from build123d import *

# Parameters (mm, degrees)
F0_R     = 9.283405223
F1_DEPTH = 25.4
F2_SIZE  = 5
F3_SIZE  = 5


with BuildPart() as f1:
    # F0 (on Top) → F1 (new body)
    with BuildSketch(Plane.XY):
        Polygon((-17.8308878342, 27.9613517337), (-33.1306848427, -1.4613259696), (-15.2997970084, -29.4226777033), (17.8308878342, -27.9613517337), (33.1306848427, 1.4613259696), (15.2997970084, 29.4226777033), align=None)
        Circle(F0_R, mode=Mode.SUBTRACT)
    extrude(amount=F1_DEPTH)

    # F2
    f2_edges = [f1.edges().sort_by_distance(p)[0] for p in [
        (-17.830888, 27.961352, 12.7),
        (15.299797, 29.422678, 12.7),
        (33.130685, 1.461326, 12.7),
        (-33.130685, -1.461326, 12.7),
        (-15.299797, -29.422678, 12.7),
        (17.830888, -27.961352, 12.7),
    ]]
    chamfer(f2_edges, length=F2_SIZE)

    # F3 (call 1 of 12: OpenCascade refuses the feature's edges together)
    f3_edges = [f1.edges().sort_by_distance(p)[0] for p in [
        (24.215241, 15.442002, 0),
    ]]
    chamfer(f3_edges, length=F3_SIZE)

    # F3#2 (call 2 of 12)
    f3_2_edges = [f1.edges().sort_by_distance(p)[0] for p in [
        (-1.265545, 28.692015, 0),
    ]]
    chamfer(f3_2_edges, length=F3_SIZE)

    # F3#3 (call 3 of 12)
    f3_3_edges = [f1.edges().sort_by_distance(p)[0] for p in [
        (24.215241, 15.442002, 25.4),
    ]]
    chamfer(f3_3_edges, length=F3_SIZE)

    # F3#4 (call 4 of 12)
    f3_4_edges = [f1.edges().sort_by_distance(p)[0] for p in [
        (-1.265545, 28.692015, 25.4),
    ]]
    chamfer(f3_4_edges, length=F3_SIZE)

    # F3#5 (call 5 of 12)
    f3_5_edges = [f1.edges().sort_by_distance(p)[0] for p in [
        (-25.480786, 13.250013, 25.4),
    ]]
    chamfer(f3_5_edges, length=F3_SIZE)

    # F3#6 (call 6 of 12)
    f3_6_edges = [f1.edges().sort_by_distance(p)[0] for p in [
        (-25.480786, 13.250013, 0),
    ]]
    chamfer(f3_6_edges, length=F3_SIZE)

    # F3#7 (call 7 of 12)
    f3_7_edges = [f1.edges().sort_by_distance(p)[0] for p in [
        (-24.215241, -15.442002, 25.4),
    ]]
    chamfer(f3_7_edges, length=F3_SIZE)

    # F3#8 (call 8 of 12)
    f3_8_edges = [f1.edges().sort_by_distance(p)[0] for p in [
        (-24.215241, -15.442002, 0),
    ]]
    chamfer(f3_8_edges, length=F3_SIZE)

    # F3#9 (call 9 of 12)
    f3_9_edges = [f1.edges().sort_by_distance(p)[0] for p in [
        (25.480786, -13.250013, 25.4),
    ]]
    chamfer(f3_9_edges, length=F3_SIZE)

    # F3#10 (call 10 of 12)
    f3_10_edges = [f1.edges().sort_by_distance(p)[0] for p in [
        (25.480786, -13.250013, 0),
    ]]
    chamfer(f3_10_edges, length=F3_SIZE)

    # F3#11 (call 11 of 12)
    f3_11_edges = [f1.edges().sort_by_distance(p)[0] for p in [
        (1.265545, -28.692015, 0),
    ]]
    chamfer(f3_11_edges, length=F3_SIZE)

    # F3#12 (call 12 of 12)
    f3_12_edges = [f1.edges().sort_by_distance(p)[0] for p in [
        (1.265545, -28.692015, 25.4),
    ]]
    chamfer(f3_12_edges, length=F3_SIZE)


solid = f1.part
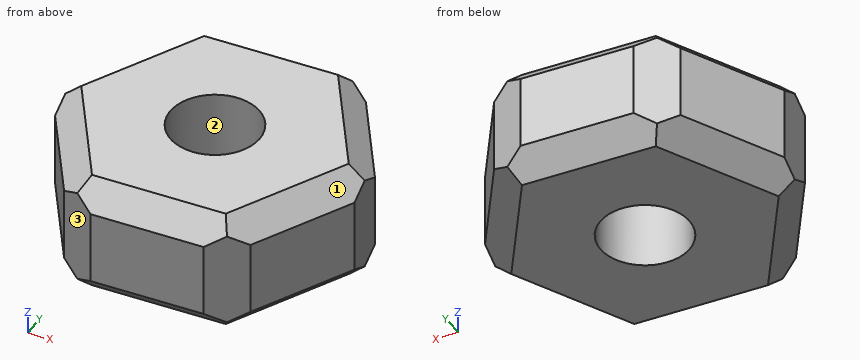
Work out the finished part from the listing and answer in its coordinate system (mm). Face numbers are marked on the shaded views. Give positions to 0.01 mm unless a question says otherwise; leave off trailing zeros. Write each loop counter-clockwise with the first axis right and the second up, starting at its lowest first coordinate (ties: lowest second). Pieces come first, ordered by that corner, then holes. Notation, with made-up numbers: (71.25, 61) - (114.25, 61) arc R5 ccw to (114.25, 69) - close; hole circle Ø2 at (2, 10.5). An arc over 180 degrees is marked (long way). One line per item, written item: value. Start each with the question number.
1. For a pull along X with two mould halves and no side action, classify the marked faces 1, 2 and 3 as +X half, -X half, draft (parallel to the pull), parting line (faces both ways), or undercut.
2. Given pin 1 (10 mm diameter, centred on x = 21, z = 9, fed in from +Y); pin 2 (10 mm diameter, centred on x = 9.5, z = 19, fed in from -Y); pin 3 (12 mm diameter, centred on y = 15.5, z = 14.5, fed in from +X), each flat-ended and moving along its own axis, determine where each tip first touches the part or whether it passes through.
3. Find section A-A (y = 8.5). Write down the section's boundary in (x, z), then the cut area to 3 significant figures.
4. Find section D-D (x = 22). Write down the section's boundary in (y, z).
5. Find section B-B (z = 13.25). Write down the section's boundary in (x, y).
6. Find section C-C (x = 1). Write down the section's boundary in (y, z), then the cut area to 3 significant figures.
7. Consider probe 1 along Y at (x, z) = (0, 5.5); probe 2 along Y at (x, z) = (0.5, 21.75); probe 3 along X at (y, z) = (3.5, 21.5). Determine where each line is inside the solid, lowest interval first.
Geometry results:
1. face 1: +X half
1. face 2: undercut
1. face 3: -X half
2. pin 1: y = 26.24
2. pin 2: y = -28.55
2. pin 3: x = 28
3. outline: (-27.95, 5) - (-22.32, 0) - (-3.73, 0) - (-3.73, 25.4) - (-22.32, 25.4) - (-27.95, 20.4) - close; (3.73, 0) - (22.71, 0) - (28.64, 5) - (28.64, 20.4) - (22.71, 25.4) - (3.73, 25.4) - close
3. area: 1,190 mm2
4. outline: (-19.94, 5) - (-9.11, 0) - (9.62, 0) - (18.92, 5) - (18.92, 20.4) - (9.62, 25.4) - (-9.11, 25.4) - (-19.94, 20.4) - close
5. outline: (-30.82, 2.97) - (-30.44, -5.68) - (-17.99, -25.21) - (-10.3, -29.2) - (12.84, -28.18) - (20.14, -23.53) - (30.82, -2.97) - (30.44, 5.68) - (17.99, 25.21) - (10.3, 29.2) - (-12.84, 28.18) - (-20.14, 23.53) - close; hole circle Ø18.57 at (0, 0)
6. outline: (-28.7, 5) - (-23.7, 0) - (-9.23, 0) - (-9.23, 25.4) - (-23.7, 25.4) - (-28.7, 20.4) - close; (9.23, 0) - (23.79, 0) - (28.79, 5) - (28.79, 20.4) - (23.79, 25.4) - (9.23, 25.4) - close
6. area: 941 mm2
7. probe 1: -28.75 to -9.28, 9.28 to 28.75
7. probe 2: -27.37 to -9.27, 9.27 to 27.42
7. probe 3: -29.31 to -8.6, 8.6 to 30.53
